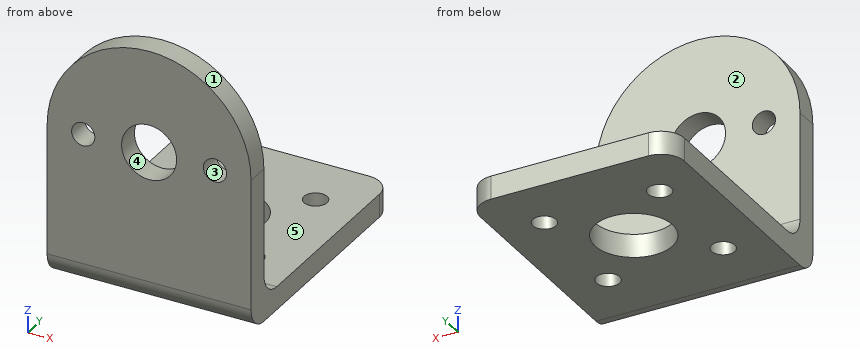
from build123d import *

# Parameters (mm, degrees)
SKETCH_R      = 3.55
SKETCH_R_2    = 1.5
PAD_DEPTH     = 3
SKETCH001_W   = 26.3
SKETCH001_H   = 3
PAD001_DEPTH  = 30
SKETCH002_R   = 5
SKETCH002_R_2 = 1.5
POCKET_DEPTH  = 3
FILLET_R      = 3
FILLET001_R   = 3


with BuildPart() as part:
    # Sketch → Pad (new body)
    with BuildSketch(Plane.XZ):
        with BuildLine():
            ThreePointArc((13.15, 0), (0, 13.15), (-13.15, 0))
            Line((-13.15, 0), (-13.15, -19.85))
            Line((13.15, -19.85), (-13.15, -19.85))
            Line((13.15, 0), (13.15, -19.85))
        make_face()
        Circle(SKETCH_R, mode=Mode.SUBTRACT)
        with Locations((8.5, 0)):
            Circle(SKETCH_R_2, mode=Mode.SUBTRACT)
        with Locations((-8.5, 0)):
            Circle(SKETCH_R_2, mode=Mode.SUBTRACT)
    extrude(amount=-PAD_DEPTH)

    # Sketch001 (on Face9 of Pad) → Pad001 (join)
    with BuildSketch(Plane(origin=(0, 3, 0), x_dir=(1, 0, 0), z_dir=(0, 1, 0))):
        with Locations((0, 18.35)):
            Rectangle(SKETCH001_W, SKETCH001_H)
    extrude(amount=PAD001_DEPTH)

    # Sketch002 (on Face7 of Pad001) → Pocket (cut)
    with BuildSketch(Plane(origin=(0, 0, -16.85), x_dir=(-1, 0, 0), z_dir=(0, 0, 1))):
        with Locations((0, -18)):
            Circle(SKETCH002_R)
        with Locations((-7.424621, -25.424621)):
            Circle(SKETCH002_R_2)
        with Locations((7.424621, -25.424621)):
            Circle(SKETCH002_R_2)
        with Locations((7.424621, -10.575379)):
            Circle(SKETCH002_R_2)
        with Locations((-7.424621, -10.575379)):
            Circle(SKETCH002_R_2)
    extrude(amount=-POCKET_DEPTH, mode=Mode.SUBTRACT)

    # Fillet
    fillet_edges = [part.edges().sort_by_distance(p)[0] for p in [
        (13.15, 33, -18.35),
        (-13.15, 33, -18.35),
    ]]
    fillet(fillet_edges, radius=FILLET_R)

    # Fillet001
    fillet001_edges = [part.edges().sort_by_distance(p)[0] for p in [
        (0, 3, -16.85),
        (0, 0, -19.85),
    ]]
    fillet(fillet001_edges, radius=FILLET001_R)


solid = part.part
Work out the finished part from the listing and answer in its coordinate system (mm). Face numbers are marked on the shaded views. A direction names the side the tool comes from. Give positions to 0.01 mm unless a question says otherwise; leave off trailing zeros. Loops run counter-clockwise (first coordinate to the right, second up) from the corner with the lowest first, then second, coordinate; pieces in that order, holes last. Notation, with made-up numbers: (62, 70) - (70, 70) arc R15 cw to (70, 74) - close; hole circle Ø7 at (50.5, 47.25). An arc over 180 degrees is marked (long way). Answer in a Markdown table with one row per item. Add a question column.
Q1. The part is cut by section A-A (y = 18). Determine the outline of the cut face in (x, z).
Q2. Determine the mould class of the marked faces 1, 2 and 3 for opening direction X: released by +X, released by -X, zero draft, split by the parting line, or undercut.
Q3. The part is cut by section C-C (z = 0.5). Determine the outline of the cut face in (x, y).
Q4. The part is cut by section D-D (z = -12.5). Determine the outline of the cut face in (x, y).
Q5. A tool of negligible diameter and unlimited length cuts with its end or side. For the marked faces 4 and 5, from which of +Z, -Z, +X, -X, +Y, -Y can it reach the whole face along a straight path? Write none if from no direction.
Q6. Consider line 1 along Y through (x, z) = (-7, -9); line 2 along Z through (x, y) = (-4, 28); line 3 along Z through (x, y) = (-8.5, 1.35). Determine where each line is inside the solid, lowest interval first.
Q7. Each of these flat-tipped pins is pushed along its axis until it touches: P1, Ø4, axis at x = 7.42, y = 25.42, coming from the +Z side; P2, Ø2, axis at x = -10, z = 2.5, coming from the +Y side. Where does it stop, or does it pass through?
Q8. The part is cut by section B-B (x = 0). Determine the outline of the cut face in (y, z), and give its area (3 significant figures).
Solution:
| question | item | result |
|---|---|---|
| 1 | outline | (-13.15, -19.85) - (-5, -19.85) - (-5, -16.85) - (-13.15, -16.85) - close; (5, -19.85) - (13.15, -19.85) - (13.15, -16.85) - (5, -16.85) - close |
| 2 | face 1 | split by the parting line |
| 2 | face 2 | zero draft |
| 2 | face 3 | undercut |
| 3 | outline | (-13.14, 0) - (-9.91, 0) - (-9.91, 3) - (-13.14, 3) - close; (-7.09, 0) - (-3.51, 0) - (-3.51, 3) - (-7.09, 3) - close; (3.51, 0) - (7.09, 0) - (7.09, 3) - (3.51, 3) - close; (9.91, 0) - (13.14, 0) - (13.14, 3) - (9.91, 3) - close |
| 4 | outline | (-13.15, 0) - (13.15, 0) - (13.15, 3) - (-13.15, 3) - close |
| 5 | face 4 | +Y, -Y |
| 5 | face 5 | +Z, +X, -X, +Y |
| 6 | line 1 | y = 0 to 3 |
| 6 | line 2 | z = -19.85 to -16.85 |
| 6 | line 3 | z = -19.36 to -1.5, 1.5 to 10.03 |
| 7 | P1 | stops at z = -16.85 |
| 7 | P2 | stops at y = 3 |
| 8 | outline | (0, -16.85) arc R3 ccw to (3, -19.85) - (13, -19.85) - (13, -16.85) - (6, -16.85) arc R3 cw to (3, -13.85) - (3, -3.55) - (0, -3.55) - close; (0, 3.55) - (3, 3.55) - (3, 13.15) - (0, 13.15) - close; (23, -19.85) - (33, -19.85) - (33, -16.85) - (23, -16.85) - close |
| 8 | area | 138 mm² |
